Work out the finished part from the listing and answer in its coordinate system (mm). Coordinates: 2 decimals unless noted, no trailing zeros. Loops run counter-clockwise (first coordinate to the right, second up) from the corner with the lowest first, then second, coordinate; pieces in that order, holes last. Notation, with made-up numbers: (61.5, 40) - (118.5, 40) arc R21 ccw to (118.5, 79) - close; hole circle Ø4 at (26.25, 72). An arc over 180 degrees is marked (long way). Write each question's results on one line, items separated by ' | '. Start each with the question number.
Item 1: Section C-C, the plane y = 8.25 is taken. Write down the section's boundary in (x, z), plus the area to 3 significant figures.
Item 2: Each of these flat-tipped pins is pushed along its axis until it touches: pin 1 Ø1.5 at (y, z) = (1, -56.5) entering from -X; pin 2 Ø6 at (x, y) = (-58, 6) entering from +Z; pin 3 Ø21 at (x, z) = (-35, -35) entering from -Y; pin 4 Ø1.5 at (x, y) = (49.5, 1.5) entering from +Z. Where does it stop, or does it pass through?
Item 3: Section A-A, the plane z = -35 is taken. Write down the section's boundary in (x, y).
Item 4: Consider probe 1 along X at (y, z) = (5.25, -35); probe 2 along Z at (x, y) = (-27.5, 6.25); probe 3 along X at (y, z) = (7.5, 34). Determine where each line is inside the solid, lowest interval first. Write a range as [from, to].
Item 5: Section B-B, the plane x = -35 is taken. Write down the section's boundary in (y, z), plus the area to 3 significant figures.
Item 6: Section D-D, the plane x = -65 is taken. Write down the section's boundary in (y, z).
Item 7: For a pull along Z with two mould halves and no side action, classify faces 1 (the face through (72.504, 4.93, -43.24)), 2 (the face through (-17, 10, 1)), 3 (the face through (-1.014, 4.93, -70.758)) as +Z half, -Z half, draft (parallel to the pull), parting line (faces both ways), or undercut.
from build123d import *

# Parameters (mm, degrees)
BOSS_EXTRUDE1_DEPTH = 10
SKETCH2_R           = 13
CUT_EXTRUDE1_DEPTH  = 10
SKETCH3_R           = 15
CUT_EXTRUDE2_DEPTH  = 10


with BuildPart() as part:
    # Sketch1 → Boss-Extrude1 (new body)
    with BuildSketch(Plane(origin=(0, 0, 0), x_dir=(1, 0, 0), z_dir=(0, 1, 0))):
        with BuildLine():
            ThreePointArc((-14.287102681, 75.958258112), (-0.806955409, 70.759221722), (12.551119215, 76.264327736))
            ThreePointArc((12.551119215, 76.264327736), (27.96684553, 79.652976213), (37.880471551, 67.370974118))
            ThreePointArc((37.880471551, 67.370974118), (44.864987287, 54.723409538), (58.636480059, 50.354160551))
            ThreePointArc((58.636480059, 50.354160551), (72.623792794, 43.040978017), (72.32335215, 27.260062589))
            ThreePointArc((72.32335215, 27.260062589), (69.544103812, 13.081905848), (77.285180212, 0.882722021))
            ThreePointArc((77.285180212, 0.882722021), (83.299260286, -13.71037214), (72.925332493, -25.606135188))
            ThreePointArc((72.925332493, -25.606135188), (61.682761267, -34.680766977), (59.771285614, -49.001751954))
            ThreePointArc((59.771285614, -49.001751954), (54.998078122, -64.046486799), (39.404739288, -66.490937729))
            ThreePointArc((39.404739288, -66.490937729), (24.959369198, -66.2159235), (14.289742194, -75.957761595))
            ThreePointArc((14.289742194, -75.957761595), (0.962683969, -84.414538487), (-12.553769364, -76.263891543))
            ThreePointArc((-12.553769364, -76.263891543), (-23.442789112, -66.767913509), (-37.878130411, -67.37229041))
            ThreePointArc((-37.878130411, -67.37229041), (-53.523160712, -65.284089454), (-58.638229812, -50.352122925))
            ThreePointArc((-58.638229812, -50.352122925), (-60.875805858, -36.078454745), (-72.322404829, -27.262575782))
            ThreePointArc((-72.322404829, -27.262575782), (-82.964923652, -15.606489414), (-77.285210839, -0.880036389))
            ThreePointArc((-77.285210839, -0.880036389), (-69.824356485, 11.492513962), (-72.926222253, 25.603601044))
            ThreePointArc((-72.926222253, 25.603601044), (-73.586476763, 41.37356047), (-59.769582785, 49.003828954))
            ThreePointArc((-59.769582785, 49.003828954), (-46.101314701, 53.686007661), (-39.4070498, 66.489568389))
            ThreePointArc((-39.4070498, 66.489568389), (-29.776099574, 78.994461594), (-14.287102681, 75.958258112))
        make_face()
    extrude(amount=BOSS_EXTRUDE1_DEPTH)

    # Sketch2 → Cut-Extrude1 (cut)
    with BuildSketch(Plane(origin=(0, 10, 0), x_dir=(-1, 0, 0), z_dir=(0, 1, 0))):
        with Locations(Location((-35, 35, 0), (0, 0, 90))):
            Circle(SKETCH2_R)
        with Locations(Location((35, 35, 0), (0, 0, 90))):
            Circle(SKETCH2_R)
        with Locations(Location((35, -35, 0), (0, 0, 90))):
            Circle(SKETCH2_R)
        with Locations(Location((-35, -35, 0), (0, 0, 90))):
            Circle(SKETCH2_R)
    extrude(amount=-CUT_EXTRUDE1_DEPTH, mode=Mode.SUBTRACT)

    # Sketch3 → Cut-Extrude2 (cut)
    with BuildSketch(Plane(origin=(0, 10, 0), x_dir=(1, 0, 0), z_dir=(0, 1, 0))):
        with Locations(Location((0, 0, 0), (0, 0, 270))):
            Circle(SKETCH3_R)
    extrude(amount=-CUT_EXTRUDE2_DEPTH, mode=Mode.SUBTRACT)


solid = part.part
Answer key:
1) outline: (-77.29, 0.88) arc R19.5 cw to (-72.93, -25.6) arc R15 ccw to (-59.77, -49) arc R19.5 cw to (-39.41, -66.49) arc R15 ccw to (-14.29, -75.96) arc R19.5 cw to (12.55, -76.26) arc R15 ccw to (37.88, -67.37) arc R19.5 cw to (58.64, -50.35) arc R15 ccw to (72.32, -27.26) arc R19.5 cw to (77.29, -0.88) arc R15 ccw to (72.93, 25.61) arc R19.5 cw to (59.77, 49) arc R15 ccw to (39.4, 66.49) arc R19.5 cw to (14.29, 75.96) arc R15 ccw to (-12.55, 76.26) arc R19.5 cw to (-37.88, 67.37) arc R15 ccw to (-58.64, 50.35) arc R19.5 cw to (-72.32, 27.26) arc R15 ccw to start; hole circle Ø26 at (-35, -35); hole circle Ø26 at (-35, 35); hole circle Ø30 at (0, 0); hole circle Ø26 at (35, -35); hole circle Ø26 at (35, 35) | area: 16,100 mm^2
2) pin 1: stops at x = -44.03 | pin 2: stops at z = 63.9 | pin 3: passes through | pin 4: stops at z = 67.25
3) outline: (-75.48, 0) - (-48, 0) - (-48, 10) - (-75.48, 10) - close; (-22, 0) - (22, 0) - (22, 10) - (-22, 10) - close; (48, 0) - (74.71, 0) - (74.71, 10) - (48, 10) - close
4) probe 1: x = [-75.48, -48], [-22, 22], [48, 74.71] | probe 2: z = [-79.65, -45.62], [-24.38, 24.38], [45.62, 65.82] | probe 3: x = [-62.3, -47.96], [-22.04, 22.04], [47.96, 62.08]
5) outline: (0, -75.66) - (10, -75.66) - (10, -48) - (0, -48) - close; (0, -22) - (10, -22) - (10, 22) - (0, 22) - close; (0, 48) - (10, 48) - (10, 66.34) - (0, 66.34) - close | area: 900 mm^2
6) outline: (0, -48.33) - (10, -48.33) - (10, 31.18) - (0, 31.18) - close
7) face 1: undercut | face 2: draft | face 3: -Z half
